The listing builds one solid part. Answer for the finished solid, in the listing's coordinates (mm). A direction names the side the tool comes from. Round coordinates to 2 decimals unless told otherwise and drop trailing zeros. Loops run counter-clockwise (first coordinate to the right, second up) from the corner with the lowest first, then second, coordinate; pieces in that order, holes last. Notation, with made-up numbers: (-27, 65.5) - (-8, 65.5) arc R29 cw to (-8, 99.5) - close; hole circle Ø2 at (-33.5, 38.25). An arc over 180 degrees is marked (long way). One line per question, with ' | ' between items. Start each with the question number.
from build123d import *

# Parameters (mm, degrees)
SKETCH1_R           = 50
BOSS_EXTRUDE1_DEPTH = 41
SKETCH2_W           = 67
SKETCH2_H           = 30
CUT_EXTRUDE1_DEPTH  = 41
SKETCH3_R           = 100
BOSS_EXTRUDE2_DEPTH = 100


with BuildPart() as part:
    # Sketch1 → Boss-Extrude1 (new body)
    with BuildSketch(Plane.XY):
        Circle(SKETCH1_R)
    extrude(amount=BOSS_EXTRUDE1_DEPTH)

    # Sketch2 → Cut-Extrude1 (cut)
    with BuildSketch(Plane.XY.offset(41)):
        Rectangle(SKETCH2_W, SKETCH2_H)
    extrude(amount=-CUT_EXTRUDE1_DEPTH, mode=Mode.SUBTRACT)

    # Sketch3 → Boss-Extrude2 (add)
    with BuildSketch(Plane(origin=(0, 0, 0), x_dir=(-1, 0, 0), z_dir=(0, 0, -1))):
        Circle(SKETCH3_R)
    extrude(amount=BOSS_EXTRUDE2_DEPTH)


solid = part.part
(1) Find section A-A on x = 0. Write down the section's boundary in (y, z).
(2) Each of these flat-tipped pins is pushed along its axis until it touches: P1, Ø4, axis at x = -31, z = -68, coming from the +Y side; P2, Ø1.5, axis at x = 74.5, y = 20.5, coming from the +Z side; P3, Ø10, axis at x = 26, z = -30.5, coming from the -Y side. Where does it stop, or does it pass through?
(3) Find section B-B on z = 20. Write down the section's boundary in (x, y), plus the area to 3 significant figures.
(4) Find section D-D on z = -4. Write down the section's boundary in (x, y), plus the area to 3 significant figures.
(5) Find section C-C on y = 22. Write down the section's boundary in (x, z), plus the area to 3 significant figures.
(6) Determine the mould class of faces 3 (the flat face through (46, -21, 0)), 4 (the cylindrical face through (-95.38, 30.04, -49.3)), 5 (the flat face through (33.5, 0, 21)) for opening direction Y: pulls with the +Y half, pulls with the -Y half, needs draft (parallel to the pull), parting line crosses it, or undercut.
(7) Consider L1, parallel to Z at x = 38, y = -44; L2, parallel to X at y = 3, z = 29.5; L3, parallel to X at y = 29.5, z = -21. Determine where each line is inside the solid, lowest interval first.
(8) A tool of negligible diameter and unlimited length cuts with its end or side. For faces 1 (the flat face through (-1, -22, 41)), 2 (the flat face through (0, 15, 21)), from which of +Z, -Z, +X, -X, +Y, -Y can it reach the whole face along a straight path? Write none if from no direction.
Answer below:
1) outline: (-100, -100) - (100, -100) - (100, 0) - (50, 0) - (50, 41) - (15, 41) - (15, 0) - (-15, 0) - (-15, 41) - (-50, 41) - (-50, 0) - (-100, 0) - close
2) P1: y = 95.7 | P2: z = 0 | P3: y = -97.77
3) outline: circle Ø100 at (0, 0); hole (-33.5, -15) - (33.5, -15) - (33.5, 15) - (-33.5, 15) - close | area: 5,840 mm2
4) outline: circle Ø200 at (0, 0) | area: 31,400 mm2
5) outline: (-97.55, -100) - (97.55, -100) - (97.55, 0) - (44.9, 0) - (44.9, 41) - (-44.9, 41) - (-44.9, 0) - (-97.55, 0) - close | area: 23,200 mm2
6) face 3: needs draft | face 4: parting line crosses it | face 5: undercut
7) L1: -100 to 0 | L2: -49.91 to -33.5, 33.5 to 49.91 | L3: -95.55 to 95.55
8) face 1: +Z, +X, -X, +Y, -Y | face 2: +Z
